For this review, take the finished solid that the model builds, in its own axes (mm). A direction names the side the tool comes from. Give positions to 0.01 mm unless a question says otherwise; leave off trailing zeros. Write each loop counter-clockwise with the first axis right and the second up, starting at its lowest first coordinate (ties: lowest second). Pieces come first, ordered by that corner, then holes. Notation, with made-up numbers: M 46.5,36.25 L 74.5,36.25 A23 ccw 74.5,58.25 Z; hole C 18,-24 d10. An arc over 180 degrees is marked long. Answer as a JSON object with one key per item and string values. Group by question number.
```python
from build123d import *

# Parameters (mm, degrees)
F1_ANGLE = 90
F2_R     = 10


with BuildPart() as f1:
    # F0 (on Front) → F1 (revolve)
    with BuildSketch(Plane.XZ):
        Polygon((700.6, 35.9), (0, 35.9), (0, 24.079584), (0, 0), (750, 0), (750, 26.5), (710, 26.5), align=None)
    revolve(axis=Axis((375, 0, 0), (1, 0, 0)), revolution_arc=F1_ANGLE)

    # F2
    f2_edges = [f1.edges().sort_by_distance(p)[0] for p in [
        (710, -18.73833, 18.73833),
    ]]
    fillet(f2_edges, radius=F2_R)


solid = f1.part
```
Item 1: Machinability: for faces 1 (the cylindrical face through (731.82, -18.531, 18.943)), 2 (the flat face through (370, 0, 18)), which of the approach directions +Z, -Z, +X, -X, +Y, -Y give a long, thin tool a straight path to every point of the face, cutting with its end or side? Answer none if there is none.
Item 2: To check wall thickness, follow probe 1 along Y at (x, z) = (426.5, 24); probe 2 along Z at (x, y) = (108.5, -21.5); probe 3 along X at (y, z) = (-32, 14). State the ranges of each line that lie inside material, in increasing order.
Item 3: Consider section A-A (x = 121). Give the boundary of the cut face in (y, z), plus the area to 3 significant figures.
Item 4: Insertion check: P1, Ø3, axis at x = 238.5, z = 10, coming from the -Y side; P2, Ø4, axis at x = 372.5, z = 4, coming from the -Y side; P3, Ø6, axis at x = 492, z = 22.5, coming from the -Y side. Each pin has a flat end and moves straight along its axis. Give the tip position at first contact, or say it passes through.
Result set:
{
 "1": {"face 1": "+Z, +X, -Y", "face 2": "+Z, -Z, +X, -X, +Y"},
 "2": {"probe 1": "y = -26.7 to 0", "probe 2": "z = 0 to 28.75", "probe 3": "x = 0 to 701.57"},
 "3": {"outline": "M -35.9,0 L 0,0 L 0,35.9 A35.9 ccw Z", "area": "1,010 mm^2"},
 "4": {"P1": "stops at y = -34.88", "P2": "stops at y = -35.84", "P3": "stops at y = -30.14"}
}
